Can you work these out from the model? Positions are in its coordinate system, mm. A direction names the side the tool comes from. Coordinates: 2 decimals unless noted, no trailing zeros. Order: outer loops, then holes, each group sorted by start corner. A loop starts at its lowest first (then second) coordinate and runs counter-clockwise, first axis right, second up. Notation, with made-up numbers: (14.5, 24.25) -> (40.5, 24.25) arc R23 cw to (40.5, 45.25) -> close; hole circle Ø10 at (67, 41). An arc over 180 degrees is marked (long way). Answer in a Markdown table with one row per item.
```python
from build123d import *

# Parameters (mm, degrees)
SKETCH1_R                = 1.5
BOSS_EXTRUDE1_DEPTH      = 1
SKETCH2_W                = 4.5
SKETCH2_H                = 8
BOSS_EXTRUDE2_DEPTH      = 3
BOSS_EXTRUDE3_DEPTH      = 7
BOSS_EXTRUDE4_DEPTH      = 0.5
BOSS_EXTRUDE4_DEPTH_BACK = 6.5
SKETCH5_W                = 2.5
SKETCH5_H                = 6.5
SKETCH5_W_2              = 2
SKETCH5_H_2              = 4
BOSS_EXTRUDE5_DEPTH      = 1


with BuildPart() as part:
    # Sketch1 → Boss-Extrude1 (new body)
    with BuildSketch(Plane(origin=(0, 0, 0), x_dir=(0, 1, 0), z_dir=(0, 0, 1))):
        with BuildLine():
            Line((-9, 11), (9, 11))
            ThreePointArc((9, 11), (10.414213562, 10.414213562), (11, 9))
            Line((11, 9), (11, -9))
            ThreePointArc((11, -9), (10.414213562, -10.414213562), (9, -11))
            Line((9, -11), (-9, -11))
            ThreePointArc((-9, -11), (-10.414213562, -10.414213562), (-11, -9))
            Line((-11, -9), (-11, 9))
            ThreePointArc((-11, 9), (-10.414213562, 10.414213562), (-9, 11))
        make_face()
        with Locations(Location((-7.75, 8.5, 0), (0, 0, 270))):
            Circle(SKETCH1_R, mode=Mode.SUBTRACT)
        with Locations(Location((7.75, 8.5, 0), (0, 0, 270))):
            Circle(SKETCH1_R, mode=Mode.SUBTRACT)
    extrude(amount=BOSS_EXTRUDE1_DEPTH)

    # Sketch2 → Boss-Extrude2 (add)
    with BuildSketch(Plane.XY.offset(1)):
        with Locations((-8.75, 0)):
            Rectangle(SKETCH2_W, SKETCH2_H)
    extrude(amount=BOSS_EXTRUDE2_DEPTH)

    # Sketch3 → Boss-Extrude3 (add)
    with BuildSketch(Plane.XY.offset(1)):
        with BuildLine():
            Line((7, 7.5), (5.196152423, 7.5))
            ThreePointArc((5.196152423, 7.5), (-6, 4.5), (5.196152423, 1.5))
            Line((5.196152423, 1.5), (7, 1.5))
            Line((7, 1.5), (7, 7.5))
        make_face()
    extrude(amount=BOSS_EXTRUDE3_DEPTH)

    # Sketch4 → Boss-Extrude4 (add, two sides: drawn at the far end of the back side and taken through both)
    with BuildSketch(Plane.YZ.offset(11).offset(-BOSS_EXTRUDE4_DEPTH_BACK)):
        with BuildLine():
            Line((-9.5, 4.5), (-2.5, 4.5))
            ThreePointArc((-2.5, 4.5), (-1.792893219, 4.207106781), (-1.5, 3.5))
            Line((-1.5, 3.5), (-1.5, 2))
            ThreePointArc((-1.5, 2), (-1.792893219, 1.292893219), (-2.5, 1))
            Line((-2.5, 1), (-9.5, 1))
            ThreePointArc((-9.5, 1), (-10.207106781, 1.292893219), (-10.5, 2))
            Line((-10.5, 2), (-10.5, 3.5))
            ThreePointArc((-10.5, 3.5), (-10.207106781, 4.207106781), (-9.5, 4.5))
        make_face()
    extrude(amount=BOSS_EXTRUDE4_DEPTH + BOSS_EXTRUDE4_DEPTH_BACK)

    # Sketch5 → Boss-Extrude5 (add)
    with BuildSketch(Plane.XY.offset(1)):
        with Locations((9.25, 4.25)):
            Rectangle(SKETCH5_W, SKETCH5_H)
        with Locations((11.5, 4.25)):
            Rectangle(SKETCH5_W_2, SKETCH5_H_2)
    extrude(amount=BOSS_EXTRUDE5_DEPTH)


solid = part.part
```
(1) I need wall thicknesses on line 1 (Y direction, x = -8.5, z = 0.3); line 2 (X direction, y = -3, z = 3.25); line 3 (Y direction, x = 6, z = 2). Which ranges of each line are inside material? Lowest first, please. Write a range as [from, to].
Response values:
| item | result |
|---|---|
| line 1 | [-11, -9.25], [-6.25, 6.25], [9.25, 11] |
| line 2 | [-11, -6.5], [4.5, 11.5] |
| line 3 | [-10.5, -1.5], [1.5, 7.5] |
(2) Suppose I cut it at D-D (z = 1.5). Please give me the cut outline in (x, y).
Response values:
| item | result |
|---|---|
| outline | (-11, -4) -> (-6.5, -4) -> (-6.5, 4) -> (-11, 4) -> close; (4.5, -10.37) -> (11.5, -10.37) -> (11.5, -1.63) -> (4.5, -1.63) -> close; (5.2, 1.5) -> (7, 1.5) -> (7, 7.5) -> (5.2, 7.5) arc R6 ccw (long way) to start; (8, 1) -> (10.5, 1) -> (10.5, 2.25) -> (12.5, 2.25) -> (12.5, 6.25) -> (10.5, 6.25) -> (10.5, 7.5) -> (8, 7.5) -> close |
(3) Will these pins go through, and if not, where does the flat tip stop? pin 1 Ø0.8 at (x, z) = (9, 1.5) entering from -Y (3 decimals); pin 2 Ø2 at (y, z) = (3, 3.5) entering from +X; pin 3 Ø0.9 at (y, z) = (0.5, 2.5) entering from +X.
Response values:
| item | result |
|---|---|
| pin 1 | y = -10.495 |
| pin 2 | x = 7 |
| pin 3 | x = 4.84 |
(4) Suppose I cut it at B-B (x = -8.5). Please give me the cut outline in (y, z).
Response values:
| item | result |
|---|---|
| outline | (-11, 0) -> (-9.25, 0) -> (-9.25, 1) -> (-11, 1) -> close; (-6.25, 0) -> (6.25, 0) -> (6.25, 1) -> (4, 1) -> (4, 4) -> (-4, 4) -> (-4, 1) -> (-6.25, 1) -> close; (9.25, 0) -> (11, 0) -> (11, 1) -> (9.25, 1) -> close |
(5) On a 3-axis mill with a long thin cutter (end or side, diameter ignored), from which of +Z, -Z, +X, -X, +Y, -Y can I reach the whole of each face in a straight line? I mean faces 1 (the flat face through (8, 4.2, 1.5)), 2 (the flat face through (9.2, 1, 1.5)), 3 (the flat face through (-6.5, 0, 2)). Say none if no direction works.
Response values:
| item | result |
|---|---|
| face 1 | +Z, +Y |
| face 2 | +Z, +X |
| face 3 | +Z, +Y, -Y |
(6) Suppose I cut it at C-C (y = -7.75). Please give me the cut outline in (x, z).
Response values:
| item | result |
|---|---|
| outline | (-11, 0) -> (-10, 0) -> (-10, 1) -> (-11, 1) -> close; (-7, 0) -> (11, 0) -> (11, 1) -> (11.5, 1) -> (11.5, 4.5) -> (4.5, 4.5) -> (4.5, 1) -> (-7, 1) -> close |
(7) Suppose I cut it at A-A (z = 3). Please give me the cut outline in (x, y).
Response values:
| item | result |
|---|---|
| outline | (-11, -4) -> (-6.5, -4) -> (-6.5, 4) -> (-11, 4) -> close; (4.5, -10.5) -> (11.5, -10.5) -> (11.5, -1.5) -> (4.5, -1.5) -> close; (5.2, 1.5) -> (7, 1.5) -> (7, 7.5) -> (5.2, 7.5) arc R6 ccw (long way) to start |
(8) We'd pull the mould along Y, two halves only. Please class faces 4 (the flat face through (11.5, 6.25, 1.5)), 5 (the flat face through (-9, -4, 2)), 6 (the flat face through (6, 1.5, 4)), 7 (the cylindrical face through (7.951, -1.801, 4.215)): +Y half, -Y half, draft (parallel to the pull), parting line (faces both ways), or undercut.
Response values:
| item | result |
|---|---|
| face 4 | +Y half |
| face 5 | -Y half |
| face 6 | undercut |
| face 7 | undercut |
